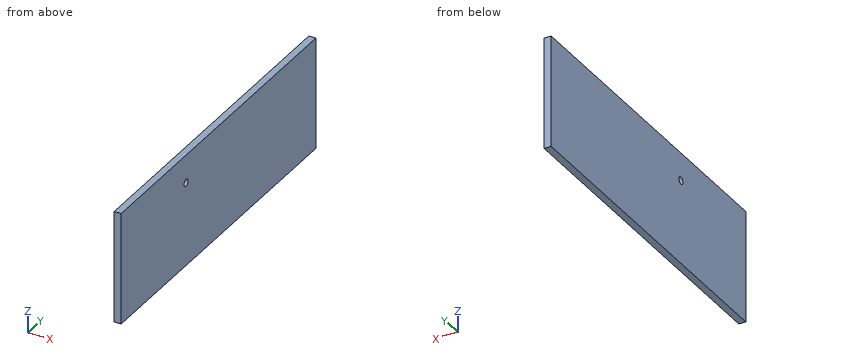
```python
from build123d import *

# Parameters (mm, degrees)
F0_W     = 152.4
F0_H     = 50.8
F2_DEPTH = 1.5875
F1_R     = 1.5875
F3_DEPTH = 1.5875


with BuildPart() as f2:
    # F0 (on Right) → F2 (new body, symmetric)
    with BuildSketch(Plane.YZ):
        Rectangle(F0_W, F0_H)
    extrude(amount=F2_DEPTH, both=True)

    # F1 (on Right) → F3 (cut, symmetric)
    with BuildSketch(Plane.YZ):
        with Locations((-25.4, 12.7)):
            Circle(F1_R)
    extrude(amount=F3_DEPTH, both=True, mode=Mode.SUBTRACT)


solid = f2.part
```
Can you work these out from the model? Positions are in its coordinate system, mm. Round coordinates to 2 decimals unless told otherwise and drop trailing zeros. Order: outer loops, then holes, each group sorted by start corner. A loop starts at its lowest first (then second) coordinate and runs counter-clockwise, first axis right, second up. Notation, with made-up numbers: (34.25, 18.5) -> (84.25, 18.5) arc R32 ccw to (84.25, 54.5) -> close; hole circle Ø1 at (50, 84). An arc over 180 degrees is marked (long way). Return JSON: item names as keys, results as strings. Group by question number.
1. I need wall thicknesses on line 1 (Z direction, x = -0.65, y = -25.4); line 2 (Z direction, x = -0.95, y = -24). Which ranges of each line are inside material? Lowest first, please. Write a range as [from, to].
2. If we section it at B-B, the plane z = 12.7: Write out the boundary of the cut face in (x, y), then the cut area to 3 significant figures.
3. If we section it at A-A, the plane y = -25.4: Write out the boundary of the cut face in (x, z).
Output values:
{
 "1": {"line 1": "[-25.4, 11.11], [14.29, 25.4]", "line 2": "[-25.4, 11.95], [13.45, 25.4]"},
 "2": {"outline": "(-1.59, -76.2) -> (1.59, -76.2) -> (1.59, -26.99) -> (-1.59, -26.99) -> close; (-1.59, -23.81) -> (1.59, -23.81) -> (1.59, 76.2) -> (-1.59, 76.2) -> close", "area": "474 mm²"},
 "3": {"outline": "(-1.59, -25.4) -> (1.59, -25.4) -> (1.59, 11.11) -> (-1.59, 11.11) -> close; (-1.59, 14.29) -> (1.59, 14.29) -> (1.59, 25.4) -> (-1.59, 25.4) -> close"}
}
